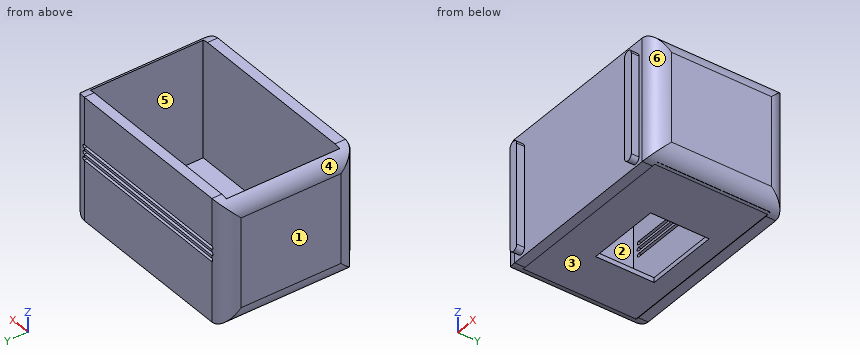
```python
from build123d import *

# Parameters (mm, degrees)
IZIM1_W                     = 121.550964813
IZIM1_H                     = 79.400227015
IZIM1_W_2                   = 108.562656073
IZIM1_H_2                   = 67.392167991
Y_KSEKLIK_EKSTR_ZYON1_DEPTH = 73.164910278
IZIM2_W                     = 108.665778405
IZIM2_H                     = 2.839609685
Y_KSEKLIK_EKSTR_ZYON3_DEPTH = 67.31
IZIM4_W                     = 43.769026383
IZIM4_H                     = 34.779664875
KES_EKSTR_ZYON3_DEPTH       = 51.308
RADYUS1_R                   = 10
RADYUS2_R                   = 10
KES_EKSTR_ZYON6_DEPTH       = 25.4
Y_KSEKLIK_EKSTR_ZYON4_DEPTH = 4.572


with BuildPart() as part:
    # Çizim1 → Yükseklik-Ekstrüzyon1 (new body)
    with BuildSketch(Plane.XY):
        with Locations((3.983010787, 3.063280364)):
            Rectangle(IZIM1_W, IZIM1_H)
        with Locations((3.860479571, 3.185811577)):
            Rectangle(IZIM1_W_2, IZIM1_H_2, mode=Mode.SUBTRACT)
    extrude(amount=Y_KSEKLIK_EKSTR_ZYON1_DEPTH)

    # Çizim2 → Yükseklik-Ekstrüzyon3 (add)
    with BuildSketch(Plane(origin=(0, -30.510272418, 0), x_dir=(1, 0, 0), z_dir=(0, 1, 0))):
        with Locations((3.70835341, -1.557090266)):
            Rectangle(IZIM2_W, IZIM2_H)
    extrude(amount=Y_KSEKLIK_EKSTR_ZYON3_DEPTH)

    # Çizim4 → Kes-Ekstrüzyon3 (cut)
    with BuildSketch(Plane(origin=(0, 0, 0.137285424), x_dir=(-1, 0, 0), z_dir=(0, 0, -1))):
        with Locations((-2.08713858, 8.765719608)):
            Rectangle(IZIM4_W, IZIM4_H)
    extrude(amount=-KES_EKSTR_ZYON3_DEPTH, mode=Mode.SUBTRACT)

    # Radyus1
    # the kernel refuses this fillet: 10 mm, written as the material it takes off along each edge
    with BuildSketch(Plane(origin=(64.758493193, -36.636833144, -25), x_dir=(0, 1, 0), z_dir=(0, 0, 1)), Plane(origin=(64.758493193, 42.763393871, -25), x_dir=(-1, 0, 0), z_dir=(0, 0, 1))) as radyus1_piece_1:
        with BuildLine():
            CenterArc((RADYUS1_R, RADYUS1_R), RADYUS1_R, 180, 90)
            Line((0, RADYUS1_R), (0, 0))
            Line((0, 0), (RADYUS1_R, 0))
        make_face()
    extrude(amount=123.164910278, mode=Mode.SUBTRACT)
    with BuildSketch(Plane(origin=(64.758493193, 67.763393871, 73.164910278), x_dir=(0, 0, -1), z_dir=(0, -1, 0))) as radyus1_piece_2:
        with BuildLine():
            CenterArc((RADYUS1_R, -RADYUS1_R), RADYUS1_R, 90, 90)
            Line((0, -RADYUS1_R), (0, 0))
            Line((0, 0), (RADYUS1_R, 0))
        make_face()
    extrude(amount=129.400227015, mode=Mode.SUBTRACT)
    with BuildSketch(Plane(origin=(64.758493193, 67.763393871, 0), x_dir=(0, 0, 1), z_dir=(0, -1, 0))) as radyus1_piece_3:
        with BuildLine():
            CenterArc((RADYUS1_R, RADYUS1_R), RADYUS1_R, 180, 90)
            Line((0, RADYUS1_R), (0, 0))
            Line((0, 0), (RADYUS1_R, 0))
        make_face()
    extrude(amount=129.400227015, mode=Mode.SUBTRACT)

    # Radyus2
    # the kernel refuses this fillet: 10 mm, written as the material it takes off along each edge
    with BuildSketch(Plane(origin=(-56.79247162, 42.763393871, -25), x_dir=(1, 0, 0), z_dir=(0, 0, 1)), Plane(origin=(-56.79247162, -36.636833144, -25), x_dir=(0, 1, 0), z_dir=(0, 0, 1))) as radyus2_piece_1:
        with BuildLine():
            CenterArc((RADYUS2_R, -RADYUS2_R), RADYUS2_R, 90, 90)
            Line((0, -RADYUS2_R), (0, 0))
            Line((0, 0), (RADYUS2_R, 0))
        make_face()
    extrude(amount=123.164910278, mode=Mode.SUBTRACT)
    with BuildSketch(Plane(origin=(-56.79247162, -61.636833144, 73.164910278), x_dir=(1, 0, 0), z_dir=(0, 1, 0))) as radyus2_piece_2:
        with BuildLine():
            CenterArc((RADYUS2_R, RADYUS2_R), RADYUS2_R, 180, 90)
            Line((0, RADYUS2_R), (0, 0))
            Line((0, 0), (RADYUS2_R, 0))
        make_face()
    extrude(amount=129.400227015, mode=Mode.SUBTRACT)
    with BuildSketch(Plane(origin=(-56.79247162, -61.636833144, 0), x_dir=(1, 0, 0), z_dir=(0, 1, 0))) as radyus2_piece_3:
        with BuildLine():
            CenterArc((RADYUS2_R, -RADYUS2_R), RADYUS2_R, 90, 90)
            Line((0, -RADYUS2_R), (0, 0))
            Line((0, 0), (RADYUS2_R, 0))
        make_face()
    extrude(amount=129.400227015, mode=Mode.SUBTRACT)

    # Çizim5 → Kes-Ekstrüzyon6 (cut)
    with BuildSketch(Plane(origin=(0, 42.763393871, 0), x_dir=(1, 0, 0), z_dir=(0, 1, 0))):
        with BuildLine():
            Line((-46.423230595, -35.751971692), (55.012749139, -35.751971692))
            ThreePointArc((55.012749139, -35.751971692), (56.029772925, -36.768995478), (55.012749139, -37.786019263))
            Line((55.012749139, -37.786019263), (-46.423230595, -37.786019263))
            ThreePointArc((-46.423230595, -37.786019263), (-47.44025438, -36.768995478), (-46.423230595, -35.751971692))
        make_face()
        with BuildLine():
            Line((-46.550358568, -42.998266165), (54.885621166, -42.998266165))
            ThreePointArc((54.885621166, -42.998266165), (55.902644952, -44.015289951), (54.885621166, -45.032313737))
            Line((54.885621166, -45.032313737), (-46.550358568, -45.032313737))
            ThreePointArc((-46.550358568, -45.032313737), (-47.567382354, -44.015289951), (-46.550358568, -42.998266165))
        make_face()
        with BuildLine():
            Line((-46.677486541, -39.438682915), (54.758493193, -39.438682915))
            ThreePointArc((54.758493193, -39.438682915), (55.775516978, -40.455706701), (54.758493193, -41.472730487))
            Line((54.758493193, -41.472730487), (-46.677486541, -41.472730487))
            ThreePointArc((-46.677486541, -41.472730487), (-47.694510327, -40.455706701), (-46.677486541, -39.438682915))
        make_face()
    extrude(amount=-KES_EKSTR_ZYON6_DEPTH, mode=Mode.SUBTRACT)

    # Çizim6 → Yükseklik-Ekstrüzyon4 (add)
    with BuildSketch(Plane(origin=(0, -36.636833144, 0), x_dir=(-1, 0, 0), z_dir=(0, -1, 0))):
        with BuildLine():
            Line((-46.87100271, -4.227005014), (-46.87100271, -64.014742354))
            ThreePointArc((-46.87100271, -64.014742354), (-49.504404567, -66.64814421), (-52.137806423, -64.014742354))
            Line((-52.137806423, -64.014742354), (-52.137806423, -4.227005014))
            ThreePointArc((-52.137806423, -4.227005014), (-49.504404567, -1.593603158), (-46.87100271, -4.227005014))
        make_face()
        with BuildLine():
            Line((44.301980946, -4.525434052), (44.301980946, -64.313171393))
            ThreePointArc((44.301980946, -64.313171393), (41.66857909, -66.946573249), (39.035177234, -64.313171393))
            Line((39.035177234, -64.313171393), (39.035177234, -4.525434052))
            ThreePointArc((39.035177234, -4.525434052), (41.66857909, -1.892032196), (44.301980946, -4.525434052))
        make_face()
    extrude(amount=Y_KSEKLIK_EKSTR_ZYON4_DEPTH)


solid = part.part
```
Model file for the job. Use its own axes, mm. Face numbers are marked on the shaded views. A direction names the side the tool comes from. Coordinates: 2 decimals unless noted, no trailing zeros. Loops run counter-clockwise (first coordinate to the right, second up) from the corner with the lowest first, then second, coordinate; pieces in that order, holes last. Notation, with made-up numbers: M 12,3 L 17,3 A19 cw 17,40 Z; hole C -7,-21.5 d1. An arc over 180 degrees is marked long. Use CSV: the item, a comma, the result in double quotes. Start each with the question number.
1. Band-saw the part on D-D, the plane x = -4. List the corners of the cut face in (y, z).
2. Two-plate mould, pull along X, no slides. Class the marked faces 3, 4, 5 and 6: pulls with the +X half, pulls with the -X half, needs draft (parallel to the pull), parting line crosses it, or undercut.
3. Tool access for the marked faces 1 and 2: list every direction of +Z, -Z, +X, -X, +Y, -Y with a clear straight run to the whole face (end or side of a thin tool).
4. Band-saw the part on A-A, the plane y = 14.5. List the corners of the cut face in (x, z), then the cut area to 3 significant figures.
5. Flat gauge pins, fed straight in: pin 1 (4 mm diameter, centred on x = -35.5, y = 20, fed in from -Z); pin 2 (10 mm diameter, centred on x = 33, y = 32, fed in from -Z); pin 3 (1.4 mm diameter, centred on y = -38, z = 24, fed in from +X); pin 4 (5 mm diameter, centred on x = -16, y = 3.5, fed in from -Z). Where does each tip first touch, or does it go through?
6. Band-saw the part on B-B, the plane z = 59. List the corners of the cut face in (x, y).
7. Probe probe 1 along Y at (x, z) = (-24.5, 64); probe 2 along X at (y, z) = (-5.5, 53.5); probe 3 along Z at (x, y) = (41.5, -24.5). List the from-to ranges inside material, lowest first. Write a range as [from, to].
8. Band-saw the part on C-C, the plane x = 42. List the corners of the cut face in (y, z).
Entries:
1,outline,"M -36.64,0 L -30.51,0 L -30.51,0.14 L -8.62,0.14 L -8.62,2.98 L -30.51,2.98 L -30.51,73.16 L -36.64,73.16 Z; M 26.16,0.14 L 36.8,0.14 L 36.8,2.98 L 26.16,2.98 Z; M 36.88,0 L 42.76,0 L 42.76,35.75 L 36.88,35.75 Z; M 36.88,37.79 L 42.76,37.79 L 42.76,39.44 L 36.88,39.44 Z; M 36.88,41.47 L 42.76,41.47 L 42.76,43 L 36.88,43 Z; M 36.88,45.03 L 42.76,45.03 L 42.76,73.16 L 36.88,73.16 Z"
2,face 3,"needs draft"
2,face 4,"pulls with the -X half"
2,face 5,"undercut"
2,face 6,"pulls with the +X half"
3,face 1,"+Z, -Z, -X, +Y, -Y"
3,face 2,"+Z"
4,outline,"M -56.79,10 A10 ccw -48.44,0.14 L -19.8,0.14 L -19.8,2.98 L -50.42,2.98 L -50.42,72.48 A10 ccw -56.79,63.16 Z; M 23.97,0.14 L 56.41,0.14 A10 ccw 58.04,0.55 L 58.04,2.98 L 23.97,2.98 Z; M 58.14,0.59 A10 ccw 64.76,10 L 64.76,63.16 A10 ccw 58.14,72.58 Z"
4,area,"1,050 mm2"
5,pin 1,"stops at z = 0.14"
5,pin 2,"stops at z = 0"
5,pin 3,"stops at x = 52.14"
5,pin 4,"passes through"
6,outline,"M -56.79,-26.64 A10 ccw -46.79,-36.64 L -44.3,-36.64 L -44.3,-41.21 L -39.04,-41.21 L -39.04,-36.64 L 46.87,-36.64 L 46.87,-41.21 L 52.14,-41.21 L 52.14,-36.64 L 54.76,-36.64 A10 ccw 64.76,-26.64 L 64.76,32.76 A10 ccw 54.76,42.76 L -46.79,42.76 A10 ccw -56.79,32.76 Z; hole M -50.42,-30.51 L 58.14,-30.51 L 58.14,36.88 L -50.42,36.88 Z"
7,probe 1,"y = [-36.64, -30.51], [36.88, 42.76]"
7,probe 2,"x = [-56.79, -50.42], [58.14, 64.76]"
7,probe 3,"z = [0.14, 2.98]"
8,outline,"M -36.64,0 L -30.51,0 L -30.51,0.14 L 36.8,0.14 L 36.8,2.98 L -30.51,2.98 L -30.51,73.16 L -36.64,73.16 Z; M 36.88,0 L 42.76,0 L 42.76,35.75 L 36.88,35.75 Z; M 36.88,37.79 L 42.76,37.79 L 42.76,39.44 L 36.88,39.44 Z; M 36.88,41.47 L 42.76,41.47 L 42.76,43 L 36.88,43 Z; M 36.88,45.03 L 42.76,45.03 L 42.76,73.16 L 36.88,73.16 Z"
